For this review, take the finished solid that the model builds, in its own axes (mm). A direction names the side the tool comes from. Give positions to 0.01 mm unless a question says otherwise; leave off trailing zeros. Write each loop counter-clockwise with the first axis right and the second up, starting at its lowest first coordinate (ties: lowest second). Pieces come first, ordered by that corner, then holes. Notation, with made-up numbers: (69, 62.25) -> (124, 62.25) arc R13 cw to (124, 78.25) -> close; hole circle Ø3 at (63, 62). An arc over 180 degrees is marked (long way). Return JSON: item names as keys, results as strings.
from build123d import *

# Parameters (mm, degrees)
CROQUIS3_W              = 50.8
CROQUIS3_H              = 6.35
CROQUIS4_W              = 50.8
CROQUIS4_H              = 6.35
SALIENTE_EXTRUIR1_DEPTH = 377
CROQUIS5_W              = 50.8
CROQUIS5_H              = 70.739551551
CORTAR_EXTRUIR1_DEPTH   = 8


with BuildPart() as part:
    # Barrer1: sweep along a curve in space
    with BuildLine() as barrer1_path:
        Line((62.290853195, 217.5, 0), (62.290853195, 217.5, 73.914551551))
        Line((62.290853195, 217.5, 73.914551551), (62.290853195, -262.5, 73.914551551))
        Line((62.290853195, -262.5, 73.914551551), (-12.709146805, -262.5, 73.914551551))
        Line((-12.709146805, -262.5, 73.914551551), (-12.709146805, 537.5, 73.914551551))
        Line((-12.709146805, 537.5, 73.914551551), (-1347.700875805, 537.5, 73.914551551))
    # Croquis3 → Barrer1 (sweep)
    with BuildSketch(Plane.XY):
        with Locations((62.290853195, 217.5)):
            Rectangle(CROQUIS3_W, CROQUIS3_H)
    sweep(path=barrer1_path.line, transition=Transition.RIGHT)

    # Croquis4 → Saliente-Extruir1 (add)
    with BuildSketch(Plane.XY.offset(77.089551551)):
        with Locations((62.290853195, 217.5)):
            Rectangle(CROQUIS4_W, CROQUIS4_H)
    extrude(amount=SALIENTE_EXTRUIR1_DEPTH)

    # Croquis5 → Cortar-Extruir1 (cut)
    with BuildSketch(Plane(origin=(0, 220.675, 0), x_dir=(1, 0, 0), z_dir=(0, 1, 0))):
        with Locations((62.290853195, -35.369775776)):
            Rectangle(CROQUIS5_W, CROQUIS5_H)
    extrude(amount=-CORTAR_EXTRUIR1_DEPTH, mode=Mode.SUBTRACT)


solid = part.part
1. Add section C-C, the plane x = -181. State the section outline as (y, z) points.
Results found:
{"outline": "(512.1, 70.74) -> (562.9, 70.74) -> (562.9, 77.09) -> (512.1, 77.09) -> close"}
2. Add section B-B, the plane z = 233. State the section outline as (x, y) points (3 decimals), plus the area to 3 significant figures.
Results found:
{"outline": "(36.891, 214.325) -> (87.691, 214.325) -> (87.691, 220.675) -> (36.891, 220.675) -> close", "area": "323 mm²"}
3. The part is to be moulded in two halves that separate along X. For faces 3 (the flat face through (36.891, -9.3, 76.9)), 4 (the flat face through (87.691, -34.8, 76.9)), 5 (the flat face through (-361, 514, 77.09)), say which applies: +X half, -X half, draft (parallel to the pull), parting line (faces both ways), or undercut.
Results found:
{"face 3": "undercut", "face 4": "+X half", "face 5": "draft"}
4. Add section A-A, the plane y = 15.5. State the section outline as (x, z) points, plus the area to 3 significant figures.
Results found:
{"outline": "(-38.11, 70.74) -> (12.69, 70.74) -> (12.69, 77.09) -> (-38.11, 77.09) -> close; (36.89, 70.74) -> (87.69, 70.74) -> (87.69, 77.09) -> (36.89, 77.09) -> close", "area": "645 mm²"}
5. For pin 1 (5 mm diameter, centred on y = 298.5, z = 74, fed in from -X); pin 2 (5 mm diameter, centred on x = -464.5, z = 75.5, fed in from -Y); pin 3 (7 mm diameter, centred on x = 22, z = 75.5, fed in from +Y), all flat-tipped, find the tip position at first contact; note any pin that passes through.
Results found:
{"pin 1": "stops at x = -38.11", "pin 2": "stops at y = 512.1", "pin 3": "stops at y = -237.1"}
6. For faces 1 (the flat face through (-368, 514, 70.74)), 2 (the flat face through (62, 214.325, 263)), list the 3-axis set-ups (+Z, -Z, +X, -X, +Y, -Y) from which the entire face can be reached by the end or side of a thin tool; tool diameter is ignored.
Results found:
{"face 1": "-Z, +X, -X, +Y, -Y", "face 2": "+Z, +X, -X, -Y"}
